from build123d import *

# Parameters (mm, degrees)
SKETCH1_R           = 150
BOSS_EXTRUDE1_DEPTH = 500
SKETCH2_W           = 150
SKETCH2_H           = 150
CUT_EXTRUDE1_DEPTH  = 544.13902456
SKETCH3_R           = 15
CUT_EXTRUDE2_DEPTH  = 544.13902456
CIRPATTERN1_COUNT   = 12
CIRPATTERN1_ANGLE   = 220


with BuildPart() as part:
    # Sketch1 → Boss-Extrude1 (new body)
    with BuildSketch(Plane.XY):
        Circle(SKETCH1_R)
    extrude(amount=-BOSS_EXTRUDE1_DEPTH)

    # Sketch2 → Cut-Extrude1 (cut, through all)
    with BuildSketch(Plane.XY):
        with Locations((75, 75)):
            Rectangle(SKETCH2_W, SKETCH2_H)
    extrude(amount=-CUT_EXTRUDE1_DEPTH, mode=Mode.SUBTRACT)

    # Sketch3 → Cut-Extrude2 (cut, through all)
    with BuildSketch(Plane.XY):
        with Locations((-38.477266124, 105.715419838)):
            Circle(SKETCH3_R)
    cut_extrude2 = extrude(amount=-CUT_EXTRUDE2_DEPTH, mode=Mode.SUBTRACT)

    # CirPattern1: Cut-Extrude2 ×12 about axis
    cirpattern1_axis = Axis((0, 0, 0), (0, 0, 1))
    for i in range(1, CIRPATTERN1_COUNT):
        add(cut_extrude2.rotate(cirpattern1_axis, i * CIRPATTERN1_ANGLE / (CIRPATTERN1_COUNT - 1)), mode=Mode.SUBTRACT)


solid = part.part
Here's how the part is built. I have some questions about the finished solid (model axes, mm). A direction names the side the tool comes from. Coordinates: 2 decimals unless noted, no trailing zeros. Write each loop counter-clockwise with the first axis right and the second up, starting at its lowest first coordinate (ties: lowest second). Pieces come first, ordered by that corner, then holes. Notation, with made-up numbers: (40.25, -29) - (66.25, -29) arc R20 ccw to (66.25, -15) - close; hole circle Ø6 at (44.25, 28.25). An arc over 180 degrees is marked (long way). Use one line per item in the form item = value.
1) Suppose I cut it at A-A, the plane z = -165. Give the number of separate pieces and of enclosed holes in the cut face, plus the area to 3 significant figures.
Solved:
separate_pieces = 1
enclosed_holes = 12
area = 44,500 mm2
2) I'm going to push flat-ended pins straight in: P1, Ø18, axis at x = 72.31, y = -86.18, coming from the +Z side; P2, Ø6, axis at y = 10, z = -83.5, coming from the +X side; P3, Ø4, axis at x = -9, z = -197.5, coming from the -Y side; P4, Ø5, axis at x = -57, z = -112, coming from the -Y side. Where does each tip first touch, or does it pass through?
Solved:
P1 = through
P2 = 0
P3 = -149.84
P4 = -139.75
3) Suppose I cut it at B-B, the plane y = -56.25. Write out the boundary of the cut face in (x, z), plus the area to 3 significant figures.
Solved:
outline = (-139.05, -500) - (-112.43, -500) - (-112.43, 0) - (-139.05, 0) - close; (-82.43, -500) - (82.43, -500) - (82.43, 0) - (-82.43, 0) - close; (112.43, -500) - (139.05, -500) - (139.05, 0) - (112.43, 0) - close
area = 109,000 mm2
4) On a 3-axis mill with a long thin cutter (end or side, diameter ignored), from which of +Z, -Z, +X, -X, +Y, -Y can I reach the whole of each face in a straight line? I mean faces 1 (the cylindrical face through (-86.17, 91.925, -246.5)), 2 (the flat face through (74, 0, -246)). Say none if no direction works.
Solved:
face_1 = +Z, -Z
face_2 = +Z, -Z, +X, +Y
5) Suppose I cut it at C-C, the plane y = 56.25. Write out the boundary of the cut face in (x, z), plus the area to 3 significant figures.
Solved:
outline = (-139.05, -500) - (-112.43, -500) - (-112.43, 0) - (-139.05, 0) - close; (-82.43, -500) - (0, -500) - (0, 0) - (-82.43, 0) - close
area = 54,500 mm2
6) Thinking about a two-plate mould opening in X: for faces 3 (the cylindrical face through (8.06, -99.85, -246.5)), 4 (the flat face through (0, 74, -246)), 5 (the flat face through (-35, 2, -500)), which applies, released by +X, released by -X, zero draft, split by the parting line, or undercut?
Solved:
face_3 = undercut
face_4 = released by +X
face_5 = zero draft
7) I need wall thicknesses on line 1 (Y direction, x = -0.5, z = -45.5); line 2 (X direction, y = -73, z = -240.5); line 3 (X direction, y = -73.5, z = -163). Which ranges of each line are inside material? Lowest first, please.
Solved:
line_1 = -150 to -127.49, -97.51 to 150
line_2 = -131.04 to -79.48, -65.15 to 65.15, 79.48 to 131.04
line_3 = -130.76 to -80.33, -64.3 to 64.3, 80.33 to 130.76
